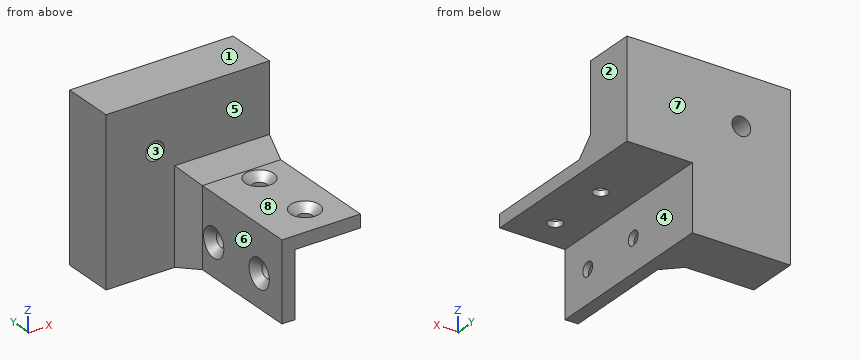
from build123d import *

# Parameters (mm, degrees)
BOSS_EXTRUDE1_DEPTH = 30
BOSS_EXTRUDE2_DEPTH = 30
SKETCH3_R           = 2.85
CUT_EXTRUDE1_DEPTH  = 67
SKETCH4_R           = 2.85
CUT_EXTRUDE2_DEPTH  = 67.627240093
SKETCH5_R           = 2.85
CUT_EXTRUDE3_DEPTH  = 67.462848717
BOSS_EXTRUDE3_DEPTH = 40
SKETCH7_R           = 2.15
CUT_EXTRUDE4_DEPTH  = 86.064681273
SKETCH8_R           = 2.15
CUT_EXTRUDE5_DEPTH  = 91.19977827
CHAMFER1_SIZE       = 2.3
CHAMFER2_SIZE       = 5
SKETCH9_W           = 30
SKETCH9_H           = 30
CUT_EXTRUDE6_DEPTH  = 76.498344353


with BuildPart() as part:
    # Sketch1 → Boss-Extrude1 (new body)
    with BuildSketch(Plane.XY):
        Polygon((10, 0), (40, -5.357142857), (38.099489796, -16), (-40, -16), (-40, 0), align=None)
    extrude(amount=BOSS_EXTRUDE1_DEPTH)

    # Sketch2 → Boss-Extrude2 (add)
    with BuildSketch(Plane.ZY.offset(40)):
        Polygon((0, 0), (-20, 0), (-50, -5.357142857), (-48.099489796, -16), (0, -16), align=None)
    extrude(amount=-BOSS_EXTRUDE2_DEPTH)

    # Sketch3 → Cut-Extrude1 (cut, through all)
    with BuildSketch(Plane(origin=(0, 0, 0), x_dir=(1, 0, 0), z_dir=(0, 1, 0))):
        with Locations(Location((-25, -15, 0), (0, 0, 180))):
            Circle(SKETCH3_R)
    extrude(amount=-CUT_EXTRUDE1_DEPTH, mode=Mode.SUBTRACT)

    # Sketch4 → Cut-Extrude2 (cut, through all)
    with BuildSketch(Plane(origin=(0.309023486, 1.73053152, 0), x_dir=(0.9844275755084806, -0.17579063848366547, 0), z_dir=(0.17579063848366547, 0.9844275755084806, 0))):
        with Locations(Location((25.081557169, -15, 0), (0, 0, 180))):
            Circle(SKETCH4_R)
    extrude(amount=-CUT_EXTRUDE2_DEPTH, mode=Mode.SUBTRACT)

    # Sketch5 → Cut-Extrude3 (cut, through all)
    with BuildSketch(Plane(origin=(0, 3.461063041, -0.618046972), x_dir=(1, 0, 0), z_dir=(0, 0.9844275755084821, -0.1757906384836575))):
        with Locations(Location((-25, 34.925832924, 0), (0, 0, 270))):
            Circle(SKETCH5_R)
    extrude(amount=-CUT_EXTRUDE3_DEPTH, mode=Mode.SUBTRACT)

    # Sketch6 → Boss-Extrude3 (add)
    with BuildSketch(Plane.XZ.offset(16)):
        Polygon((-10, 0), (-10, -20), (-14, -20), (-14, 4), (10, 4), (10, 0), align=None)
    extrude(amount=BOSS_EXTRUDE3_DEPTH)

    # Sketch7 → Cut-Extrude4 (cut, through all)
    with BuildSketch(Plane(origin=(0, 0, 0), x_dir=(-1, 0, 0), z_dir=(0, 0, -1))):
        with Locations((0, -46)):
            Circle(SKETCH7_R)
        with Locations((0, -26)):
            Circle(SKETCH7_R)
    extrude(amount=-CUT_EXTRUDE4_DEPTH, mode=Mode.SUBTRACT)

    # Sketch8 → Cut-Extrude5 (cut, through all)
    with BuildSketch(Plane(origin=(-10, 0, 0), x_dir=(0, 0, -1), z_dir=(1, 0, 0))):
        with Locations((10, -46)):
            Circle(SKETCH8_R)
        with Locations((10, -26)):
            Circle(SKETCH8_R)
    extrude(amount=-CUT_EXTRUDE5_DEPTH, mode=Mode.SUBTRACT)

    # Chamfer1
    chamfer1_edges = [part.edges().sort_by_distance(p)[0] for p in [
        (2.15, -46, 4),
        (2.15, -26, 4),
        (-14, -46, -7.85),
        (-14, -26, -7.85),
    ]]
    chamfer(chamfer1_edges, length=CHAMFER1_SIZE)

    # Chamfer2
    chamfer2_edges = [part.edges().sort_by_distance(p)[0] for p in [
        (-2, -16, 4),
        (-14, -16, -8),
    ]]
    chamfer(chamfer2_edges, length=CHAMFER2_SIZE)

    # Sketch9 → Cut-Extrude6 (cut, through all)
    with BuildSketch(Plane.XZ.offset(16)):
        with Locations((25, 15)):
            Rectangle(SKETCH9_W, SKETCH9_H)
        with Locations((-25, -35)):
            Rectangle(SKETCH9_W, SKETCH9_H)
    extrude(amount=-CUT_EXTRUDE6_DEPTH, mode=Mode.SUBTRACT)


solid = part.part
CAD build for the part. Positions are in the model's coordinates, mm. Face numbers are marked on the shaded views. A direction names the side the tool comes from. Give positions to 0.01 mm unless a question says otherwise; leave off trailing zeros. Loops run counter-clockwise (first coordinate to the right, second up) from the corner with the lowest first, then second, coordinate; pieces in that order, holes last. Notation, with made-up numbers: M -4.75,-28.75 L 41.25,-28.75 A28 cw 41.25,9.25 Z; hole C 13,-5.75 d11. An arc over 180 degrees is marked long. Answer in a Markdown table with one row per item. Add a question column.
Item 1: Band-saw the part on C-C on y = -26. Give the cut face in (x, z).
Item 2: Band-saw the part on D-D on z = 3. Give the cut face in (x, y), then the cut area to 3 significant figures.
Item 3: Drop flat-ended pins along their axis: P1, Ø5, axis at y = -46, z = -10, coming from the +X side; P2, Ø19, axis at y = -31.5, z = -14, coming from the -X side; P3, Ø12, axis at x = -1.5, y = -40, coming from the +Z side. Give the stop position or say it passes through.
Item 4: Tool access for the marked faces 4, 5, 6, 7 and 8: list every direction of +Z, -Z, +X, -X, +Y, -Y with a clear straight run to the whole face (end or side of a thin tool).
Item 5: Band-saw the part on B-B on x = -25. Give the cut face in (y, z), then the cut area to 3 significant figures.
Item 6: Band-saw the part on A-A on z = -10. Give the cut face in (x, y), then the cut area to 3 significant figures.
Item 7: Probe probe 1 along Y at (x, z) = (0, 1.1); probe 2 along Y at (x, z) = (-30, 19.5); probe 3 along Z at (x, y) = (5.5, -38). List the from-to ranges inside material, lowest first.
Item 8: Mould opens along X. For the marked faces 1, 2 and 3 say: +X half, -X half, draft (parallel to the pull), parting line (faces both ways), or undercut.
Reply:
| question | item | result |
|---|---|---|
| 1 | outline | M -14,-20 L -10,-20 L -10,-12.15 L -11.7,-12.15 L -14,-14.45 Z; M -14,-5.55 L -11.7,-7.85 L -10,-7.85 L -10,0 L -2.15,0 L -2.15,1.7 L -4.45,4 L -14,4 Z; M 2.15,0 L 10,0 L 10,4 L 4.45,4 L 2.15,1.7 Z |
| 2 | outline | M -40,-16 L -19,-16 L -14,-21 L -14,-56 L 10,-56 L 10,0 L -40,0 Z; hole C 0,-46 d6.9; hole C 0,-26 d6.9 |
| 2 | area | 1,700 mm^2 |
| 3 | P1 | stops at x = -10 |
| 3 | P2 | stops at x = -14 |
| 3 | P3 | stops at z = 4 |
| 4 | face 4 | -Z, +X, +Y, -Y |
| 4 | face 5 | +Z, -X, -Y |
| 4 | face 6 | +Z, -Z, -X, -Y |
| 4 | face 7 | +Z, -Z, +X, -X, +Y |
| 4 | face 8 | +Z, +X, -X, -Y |
| 5 | outline | M -16,-20 L 0,-20 L 0,12.15 L -16,12.15 Z; M -16,17.85 L 0,17.85 L 0,30 L -16,30 Z |
| 5 | area | 709 mm^2 |
| 6 | outline | M -40,-16 L -19,-16 L -14,-21 L -14,-21.55 L -11.7,-23.85 L -10,-23.85 L -10,0 L -40,0 Z; M -14,-56 L -10,-56 L -10,-48.15 L -11.7,-48.15 L -14,-50.45 Z; M -14,-41.55 L -11.7,-43.85 L -10,-43.85 L -10,-28.15 L -11.7,-28.15 L -14,-30.45 Z |
| 6 | area | 608 mm^2 |
| 7 | probe 1 | y = -56 to -48.15, -43.85 to -28.15, -23.85 to 0 |
| 7 | probe 2 | y = -16 to 0 |
| 7 | probe 3 | z = 0 to 4 |
| 8 | face 1 | draft |
| 8 | face 2 | +X half |
| 8 | face 3 | undercut |
